```python
from build123d import *

# Parameters (mm, degrees)
SKETCH_1_W          = 15.6
SKETCH_1_H          = 13.7
EXTRUDE_1_DEPTH     = 2
EXTRUDE_2_DEPTH     = 7.5
SKETCH_4_W          = 21.6
SKETCH_4_H          = 22.5
EXTRUDE_3_DEPTH     = 15
CHAMFER_1_SIZE      = 4
SKETCH_5_R          = 5
EXTRUDE_4_DEPTH     = 15
CUT_EXTRUDE_1_DEPTH = 0.1
HOLE_WIZARD_M3_1_D  = 2.5


with BuildPart() as part:
    # 草图1 → 凸台-拉伸1 (new body)
    with BuildSketch(Plane(origin=(0, 0, 0), x_dir=(1, 0, 0), z_dir=(0, 1, 0))):
        Rectangle(SKETCH_1_W, SKETCH_1_H)
    extrude(amount=EXTRUDE_1_DEPTH)

    # 草图3 → 凸台-拉伸2 (add)
    with BuildSketch(Plane.XZ):
        with BuildLine():
            Line((-10.8, 9.35), (10.8, 9.35))
            Line((10.8, 9.35), (10.8, 3.1))
            Line((10.8, 3.1), (13.5, 3.1))
            ThreePointArc((13.5, 3.1), (18.5, -1.9), (13.5, -6.9))
            Line((13.5, -6.9), (10.8, -6.9))
            Line((10.8, -6.9), (10.8, -13.15))
            Line((10.8, -13.15), (-10.8, -13.15))
            Line((-10.8, -13.15), (-10.8, -6.9))
            Line((-10.8, -6.9), (-13.5, -6.9))
            ThreePointArc((-13.5, -6.9), (-18.5, -1.9), (-13.5, 3.1))
            Line((-13.5, 3.1), (-10.8, 3.1))
            Line((-10.8, 3.1), (-10.8, 9.35))
        make_face()
    extrude(amount=EXTRUDE_2_DEPTH)

    # 草图4 → 凸台-拉伸3 (add)
    with BuildSketch(Plane.XZ.offset(7.5)):
        with Locations((0, -1.9)):
            Rectangle(SKETCH_4_W, SKETCH_4_H)
    extrude(amount=EXTRUDE_3_DEPTH)

    # 倒角1
    chamfer_1_edges = [part.edges().sort_by_distance(p)[0] for p in [
        (-10.8, -22.5, -1.9),
        (0, -22.5, -13.15),
        (10.8, -22.5, -1.9),
        (0, -22.5, 9.35),
    ]]
    chamfer(chamfer_1_edges, length=CHAMFER_1_SIZE)

    # 草图5 → 凸台-拉伸4 (add)
    with BuildSketch(Plane.XZ.offset(22.5)):
        with Locations(Location((0, -1.9, 0), (0, 0, 270))):
            Circle(SKETCH_5_R)
    extrude(amount=EXTRUDE_4_DEPTH)

    # 草图6 → 切除-拉伸1 (cut)
    with BuildSketch(Plane(origin=(0, 2, 0), x_dir=(1, 0, 0), z_dir=(0, 1, 0))):
        Polygon((5.326744566, -3.869583795), (-5.326744566, -3.869583795), (-5.326744566, 3.869583795), (-3.458685709, 3.869583795), (-3.458685709, 5.575202752), (3.458685709, 5.575202752), (3.458685709, 3.869583795), (5.326744566, 3.869583795), align=None)
    extrude(amount=-CUT_EXTRUDE_1_DEPTH, mode=Mode.SUBTRACT)

    # M3 螺纹孔1 (through all)
    with Locations(Plane(origin=(0, 0, 0), x_dir=(1, 0, 0), z_dir=(0, 1, 0))):
        with Locations((13.9, 1.9), (-13.9, 1.9)):
            Hole(HOLE_WIZARD_M3_1_D / 2)


solid = part.part
```
Here's how the part is built. I have some questions about the finished solid (model axes, mm). A direction names the side the tool comes from. Give positions to 0.01 mm unless a question says otherwise; leave off trailing zeros. Loops run counter-clockwise (first coordinate to the right, second up) from the corner with the lowest first, then second, coordinate; pieces in that order, holes last. Notation, with made-up numbers: (42.25, 5) -> (52.25, 5) arc R24 ccw to (52.25, 23) -> close; hole circle Ø2 at (-24.5, -4). An arc over 180 degrees is marked (long way). Use one line per item in the form item = value. Start each with the question number.
1) Imagine slicing it at B-B (z = -10.25). Please give me the cut outline in (x, y), then the cut area to 3 significant figures.
2) Which directions (+Z, -Z, +X, -X, +Y, -Y) give clear straight access to the entire face, cutting with the end or side of a thin tool? Please do faces 5 (the face through (12, -4, -6.9)), 6 (the face through (15, -7.5, -3)), 7 (the face through (-15, -7.5, -3)), 8 (the face through (-7.8, 1, 0)), 9 (the face through (7.8, 1, 0)).
3) Thinking about a two-plate mould opening in Z: for faces 1 (the face through (15.15, -3.8, -1.95)), 2 (the face through (12, -4, 3.1)), 3 (the face through (0, 1.9, -1)), 4 (the face through (-18.5, -3.7, -2)), which applies, +Z half, -Z half, draft (parallel to the pull), parting line (faces both ways), or undercut?
4) For P1, Ø3, axis at y = -29, z = -1.5, coming from the -X side; P2, Ø1, axis at y = 1, z = 3, coming from the -X side; P3, Ø3, axis at x = 13.9, z = -1.9, coming from the -Y side, each with a flat end and sliding along its axis, tell me the tip position at first contact or that it passes through.
5) Imagine slicing it at A-A (z = -1.9). Count the separate pieces of the cut face and the enclosed holes in it, then the cut area to 3 significant figures.
6) Please list where these lines run through material, in increasing order: line 1 along X through (y, z) = (-2.5, -9.75); line 2 along Y through (x, z) = (6, -3.75); line 3 along Y through (x, z) = (2.5, -7).
7) Imagine slicing it at C-C (y = -14). Please give me the cut outline in (x, z), then the cut area to 3 significant figures.
8) Imagine slicing it at D-D (x = 2). Please give me the cut outline in (y, z), then the cut area to 3 significant figures.
Check values:
q1.outline = (-10.8, -18.5) -> (-7.9, -21.4) -> (7.9, -21.4) -> (10.8, -18.5) -> (10.8, 0) -> (-10.8, 0) -> close
q1.area = 454 mm^2
q2.face_5 = -Z, +X, +Y, -Y
q2.face_6 = +Z, -Z, +X, -Y
q2.face_7 = +Z, -Z, -X, -Y
q2.face_8 = +Z, -Z, -X, +Y
q2.face_9 = +Z, -Z, +X, +Y
q3.face_1 = undercut
q3.face_2 = +Z half
q3.face_3 = undercut
q3.face_4 = parting line
q4.P1 = -5
q4.P2 = -7.8
q4.P3 = -7.5
q5.separate_pieces = 3
q5.enclosed_holes = 0
q5.area = 728 mm^2
q6.line_1 = -10.8 to 10.8
q6.line_2 = -22.5 to 2
q6.line_3 = -22.5 to 0
q7.outline = (-10.8, -13.15) -> (10.8, -13.15) -> (10.8, 9.35) -> (-10.8, 9.35) -> close
q7.area = 486 mm^2
q8.outline = (-37.5, -6.48) -> (-22.5, -6.48) -> (-22.5, -9.15) -> (-18.5, -13.15) -> (0, -13.15) -> (0, -6.85) -> (2, -6.85) -> (2, -5.58) -> (1.9, -5.58) -> (1.9, 3.87) -> (2, 3.87) -> (2, 6.85) -> (0, 6.85) -> (0, 9.35) -> (-18.5, 9.35) -> (-22.5, 5.35) -> (-22.5, 2.68) -> (-37.5, 2.68) -> close
q8.area = 654 mm^2
